Read the model definition and answer for the solid it produces. Units are mm, in the model's axes. A direction names the side the tool comes from. Coordinates: 2 decimals unless noted, no trailing zeros. Write each loop counter-clockwise with the first axis right and the second up, starting at its lowest first coordinate (ties: lowest second). Pieces come first, ordered by that corner, then holes.
from build123d import *

# Parameters (mm, degrees)
F0_R     = 0.75
F1_DEPTH = 1.1


# Not quite as in the source:
# - a feature of the source that left no trace in its solid (it failed there, or was rolled back) is left out


with BuildPart() as f1:
    # F0 (on Front) → F1 (new body)
    with BuildSketch(Plane.XZ):
        with BuildLine():
            Line((2.3143409039, -4.9458075121), (2.9332922899, -6.1348020622))
            ThreePointArc((2.9332922899, -6.1348020622), (0, 6.8), (-2.9332922899, -6.1348020622))
            Line((-2.9332922899, -6.1348020622), (-2.3143409039, -4.9458075121))
            ThreePointArc((-2.3143409039, -4.9458075121), (-2.4751182669, -3.5538688963), (-3.8270774065, -3.1856991587))
            ThreePointArc((-3.8270774065, -3.1856991587), (-4.5602291476, -3.1514585807), (-5.0725348367, -2.6258857756))
            ThreePointArc((-5.0725348367, -2.6258857756), (0, 5), (5.0725348367, -2.6258857756))
            ThreePointArc((5.0725348367, -2.6258857756), (4.5602291476, -3.1514585807), (3.8270774065, -3.1856991587))
            ThreePointArc((3.8270774065, -3.1856991587), (2.4751182669, -3.5538688963), (2.3143409039, -4.9458075121))
        make_face()
        with Locations((-3.4231044454, -4.3686217456)):
            Circle(F0_R, mode=Mode.SUBTRACT)
        with Locations((3.4231044454, -4.3686217456)):
            Circle(F0_R, mode=Mode.SUBTRACT)
    extrude(amount=F1_DEPTH)


solid = f1.part
Item 1: The part is cut by section D-D (x = 6). Give the vertices of the cut face in (y, z).
Item 2: Find the intervals of material crossed by probe 1 along Z at (x, y) = (-2.75, -0.45); probe 2 along Z at (x, y) = (-4.75, -0.5); probe 3 along X at (y, z) = (-0.25, -5.5), in increasing order.
Item 3: Determine the mould class of faces 1 (the cylindrical face through (-0.151, -0.542, 4.998)), 2 (the flat face through (-1, -1.1, 5.2)), 3 (the cylindrical face through (0.257, -0.542, 6.795)) for opening direction Z: +Z half, -Z half, draft (parallel to the pull), parting line (faces both ways), or undercut.
Item 4: The part is cut by section C-C (y = -0.25). Give the vertices of the cut face in (x, z), and give its area (3 significant figures).
Item 5: For faces 4 (the cylindrical face through (-4.551, -0.542, -3.156)), 5 (the flat face through (-1, 0, 5.2)), 6 (the flat face through (-2.63, -0.54, -5.55)), determine the directions among +Z, -Z, +X, -X, +Y, -Y from which every point of the face is accessible in a straight line to the end or side of a thin tool.
Item 6: The part is cut by section B-B (z = -0.75). Give the vertices of the cut face in (x, y), and give its area (3 significant figures).
Item 7: The part is cut by section A-A (x = 3.5). Give the vertices of the cut face in (y, z), and give its area (3 significant figures).
Answer:
1. outline: (-1.1, -3.2) - (0, -3.2) - (0, 3.2) - (-1.1, 3.2) - close
2. probe 1: z = -5.78 to -4.7, -4.04 to -3.32, 4.26 to 6.22
2. probe 2: z = -4.87 to -3.04, 2.27 to 4.87
2. probe 3: x = -4 to -2.6, 2.6 to 4
3. face 1: undercut
3. face 2: draft
3. face 3: parting line
4. outline: (-5.07, -2.63) arc R5.5 cw (long way) to (5.07, -2.63) arc R1 cw to (3.83, -3.19) arc R1.25 ccw to (2.31, -4.95) - (2.93, -6.13) arc R6.8 ccw (long way) to (-2.93, -6.13) - (-2.31, -4.95) arc R1.25 ccw to (-3.83, -3.19) arc R1 cw to start; hole circle Ø1.5 at (-3.42, -4.37); hole circle Ø1.5 at (3.42, -4.37)
4. area: 48.9 mm2
5. face 4: +Y, -Y
5. face 5: +Z, -Z, +X, -X, +Y
5. face 6: -Z, +Y, -Y
6. outline: (-6.76, -1.1) - (-5.49, -1.1) - (-5.49, 0) - (-6.76, 0) - close; (5.49, -1.1) - (6.76, -1.1) - (6.76, 0) - (5.49, 0) - close
6. area: 2.78 mm2
7. outline: (-1.1, -5.83) - (0, -5.83) - (0, -5.11) - (-1.1, -5.11) - close; (-1.1, -3.62) - (0, -3.62) - (0, -3.12) - (-1.1, -3.12) - close; (-1.1, 3.74) - (0, 3.74) - (0, 5.83) - (-1.1, 5.83) - close
7. area: 3.63 mm2
